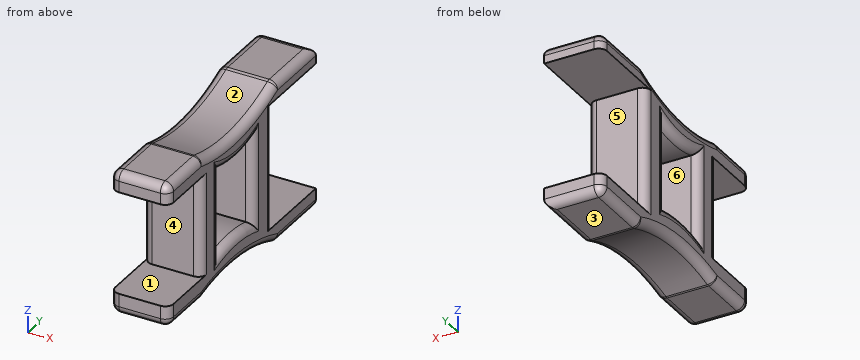
Autodesk Inventor part; units mm, degrees
ref_plane "YZ Plane" through (0, 0, 0) normal (1, 0, 0) x (0, 1, 0)
ref_plane "XZ Plane" through (0, 0, 0) normal (0, 1, 0) x (-1, 0, 0)
ref_plane "XY Plane" through (0, 0, 0) normal (0, 0, 1) x (1, 0, 0)
sketch "Sketch2" plane through (0, 0, 0) normal (1, 0, 0) x (0, 1, 0)
  line L0 (-11.003, -19.3563) -> (11.003, -19.3563)
  line L1 (11.003, -19.3563) -> (11.003, 19.3563)
  line L2 (11.003, 19.3563) -> (-11.003, 19.3563)
  line L3 (57.7702, -23.7983) -> (86.9201, -23.7983)
  line L4 (86.9201, 23.7983) -> (57.7702, 23.7983)
  line L5 (57.7702, 23.7983) -> (57.7702, -23.7983)
  line L6 (57.7702, -23.7983) -> (60.4906, -19.3563) construction
  line L7 (60.4906, 19.3563) -> (57.7702, 23.7983) construction
  line L8 (86.9201, 29.9796) -> (60.767, 29.9796)
  line L9 (86.9201, -31.153) -> (60.767, -31.153)
  line L10 (-11.003, -27.448) -> (11.003, -27.448)
  line L11 (-11.003, 26.7377) -> (11.003, 26.7377)
  arc A0 (11.003, 26.7377) -> (60.767, 29.9796) centre (31.4829, 95.932) ccw
  arc A1 (60.767, -31.153) -> (11.003, -27.448) centre (30.5123, -101.4643) ccw
  line L12 (45.6284, 16.3623) -> (45.6284, -16.3623)
  line L13 (22.3276, 16.3623) -> (22.3276, -16.3623)
  arc A2 (22.3276, 16.3623) -> (45.6284, 16.3623) centre (33.978, 54.9478) ccw
  arc A3 (45.6284, -16.3623) -> (22.3276, -16.3623) centre (33.978, -64.7297) ccw
  line L14 (-11.003, 26.7377) -> (-11.003, 19.3563)
  line L15 (-11.003, -19.3563) -> (-11.003, -27.448)
  line L16 (86.9201, 29.9796) -> (86.9201, 23.7983)
  line L17 (86.9201, -23.7983) -> (86.9201, -31.153)
  point P0 (0, 0)
extrude "Extrusion2" add sketch "Sketch2" along normal blind 22
fillet "Fillet2" radius 3.175 38 edges at (22, 73.8435, 29.9796) (11, 60.767, 29.9796) (0, 73.8435, 29.9796) (0, 36.1739, 23.9231) (22, 36.1739, 23.9231) (22, 57.7702, 0) (22, 45.6284, 0) (22, 22.3276, 0) (22, 11.003, 0) (22, 33.978, -14.9789) (22, 33.978, 14.6418) (22, 36.1954, -25.1313) (22, 73.8435, -31.153) (11, 86.9201, -31.153) (11, 86.9201, 29.9796) (11, 11.003, 26.7377) (22, 0, 26.7377) (0, 0, 26.7377) (22, 0, -27.448) (0, 73.8435, -31.153) (11, 60.767, -31.153) (0, 36.1954, -25.1313) (11, 11.003, -27.448) (0, 22.3276, 0) (0, 45.6284, 0) (0, 33.978, 14.6418) (0, 33.978, -14.9789) (0, 0, -27.448) (11, -11.003, -27.448) (11, -11.003, 26.7377) (0, 11.003, 0) (0, 57.7702, 0) (0, 86.9201, -27.4756) (0, 86.9201, 26.889) (0, -11.003, -23.4021) (0, -11.003, 23.047) (22, -11.003, 23.047) (22, -11.003, -23.4021)
properties part number "arm_mid_link2"
Could you check a few things on this model? Use its own coordinates, in mm. Face numbers are marked on the shaded views. A direction names the side the tool comes from. Coordinates: 2 decimals unless noted, no trailing zeros. Order: outer loops, then holes, each group sorted by start corner. A loop starts at its lowest first (then second) coordinate and runs counter-clockwise, first axis right, second up. Notation, with made-up numbers: (34, 82) - (74, 82) arc R23 cw to (74, 90) - close; hole circle Ø8 at (83, 25). An arc over 180 degrees is marked (long way). Answer in a Markdown table with one row per item. Add a question column.
(1) Will these pins go through, and if not, where does the flat tip stop? pin 1 (12.5 mm diameter, centred on x = 8.5, z = 6.5, fed in from -Y); pin 2 (2 mm diameter, centred on x = 14, z = 13, fed in from +Y); pin 3 (6 mm diameter, centred on y = 60.5, z = -13.5, fed in from -X).
(2) If we section it at B-B, the plane z = 13.5: Please give me the cut outline in (x, y).
(3) If we section it at D-D, the plane x = 20.5: Please give me the cut outline in (y, z), then the cut area to 3 significant figures.
(4) If we mould it in two halves opening along Z, with no side actions, what happens to the marked faces 1, 2 and 3? For each: released by +Z, released by -Z, zero draft, split by the parting line, or undercut.
(5) If we section it at A-A, the plane y = -0.5: Please give me the cut outline in (x, z).
(6) I need wall thicknesses on L1, parallel to Z at x = 3, y = 8; L2, parallel to Y at x = 14, z = 8; L3, parallel to Z at x = 18.25, y = 73.5. Which ranges of each line are inside material? Lowest first, please.
(7) On a 3-axis mill with a long thin cutter (end or side, diameter ignored), from which of +Z, -Z, +X, -X, +Y, -Y can I reach the whole of each face in a straight line? I mean the marked faces 4, 5 and 6. Say none if no direction works.
(8) If we section it at C-C, the plane x = 5.5: Please give me the cut outline in (y, z).
Results are:
| question | item | result |
|---|---|---|
| 1 | pin 1 | stops at y = 11 |
| 1 | pin 2 | stops at y = 57.77 |
| 1 | pin 3 | stops at x = 1.89 |
| 2 | outline | (0, 14.18) arc R3.17 ccw to (3.17, 11) - (18.83, 11) arc R3.17 ccw to (22, 14.18) - (22, 19.15) arc R3.17 ccw to (18.83, 22.33) - (3.17, 22.33) arc R3.17 ccw to (0, 19.15) - close; (0, 48.8) arc R3.17 ccw to (3.17, 45.63) - (18.83, 45.63) arc R3.17 ccw to (22, 48.8) - (22, 54.6) arc R3.17 ccw to (18.83, 57.77) - (3.17, 57.77) arc R3.17 ccw to (0, 54.6) - close |
| 3 | outline | (-10.53, -24.27) arc R2.7 ccw to (-7.83, -26.97) - (10.6, -26.97) arc R2.7 ccw to (11.27, -26.88) arc R77.02 cw to (60.37, -30.46) arc R2.7 ccw to (61.41, -30.68) - (85.42, -30.68) arc R3.17 ccw to (86.92, -27.98) - (86.92, -23.8) - (57.29, -23.8) - (57.29, 23.8) - (86.92, 23.8) - (86.92, 26.81) arc R3.17 ccw to (85.42, 29.5) - (61.43, 29.5) arc R2.7 ccw to (60.36, 29.28) arc R72.64 cw to (11.3, 26.15) arc R2.7 ccw to (10.55, 26.26) - (-7.83, 26.26) arc R2.7 ccw to (-10.53, 23.56) - (-10.53, 19.36) - (11.48, 19.36) - (11.48, -19.36) - (-10.53, -19.36) - close; hole (21.85, -16.97) arc R49.27 cw to (46.11, -16.97) - (46.11, 17.01) arc R39.83 cw to (21.85, 17.01) - close |
| 3 | area | 2,220 mm2 |
| 4 | face 1 | undercut |
| 4 | face 2 | released by +Z |
| 4 | face 3 | released by -Z |
| 5 | outline | (0, -24.27) arc R3.17 ccw to (3.17, -27.45) - (18.83, -27.45) arc R3.17 ccw to (22, -24.27) - (22, -19.36) - (0, -19.36) - close; (0, 19.36) - (22, 19.36) - (22, 23.56) arc R3.17 ccw to (18.83, 26.74) - (3.17, 26.74) arc R3.17 ccw to (0, 23.56) - close |
| 6 | L1 | z = -27.44 to -19.36, 19.36 to 26.73 |
| 6 | L2 | y = 11 to 22.33, 45.63 to 57.77 |
| 6 | L3 | z = -31.15 to -23.8, 23.8 to 29.98 |
| 7 | face 4 | +X, -X, -Y |
| 7 | face 5 | +X, -X, +Y |
| 7 | face 6 | +X, -X |
| 8 | outline | (-11, -24.27) arc R3.17 ccw to (-7.83, -27.45) - (10.6, -27.45) arc R3.17 ccw to (11.39, -27.35) arc R76.54 cw to (60.18, -30.9) arc R3.17 ccw to (61.41, -31.15) - (83.75, -31.15) arc R3.17 ccw to (86.92, -27.98) - (86.92, -23.8) - (57.77, -23.8) - (57.77, 23.8) - (86.92, 23.8) - (86.92, 26.81) arc R3.17 ccw to (83.75, 29.98) - (61.43, 29.98) arc R3.17 ccw to (60.17, 29.72) arc R72.16 cw to (11.43, 26.61) arc R3.17 ccw to (10.55, 26.74) - (-7.83, 26.74) arc R3.17 ccw to (-11, 23.56) - (-11, 19.36) - (11, 19.36) - (11, -19.36) - (-11, -19.36) - close; hole (22.33, -16.36) arc R49.75 cw to (45.63, -16.36) - (45.63, 16.36) arc R40.31 cw to (22.33, 16.36) - close |
